Read the model definition and answer for the solid it produces. Units are mm, in the model's axes. Round coordinates to 2 decimals unless told otherwise and drop trailing zeros. Write each loop counter-clockwise with the first axis right and the second up, starting at its lowest first coordinate (ties: lowest second). Pieces come first, ordered by that corner, then holes. Notation, with made-up numbers: (73, -10.5) - (91, -10.5) arc R26 cw to (91, 12.5) - close; hole circle Ø4 at (61, -16.75). An arc over 180 degrees is marked (long way). Use one line per item in the form item = value. Start each with the question number.
1) The part is cut by section B-B, the plane x = -173.5. Give the vertices of the cut face in (y, z).
2) The part is cut by section A-A, the plane z = 3.2. Give the vertices of the cut face in (x, y), plus the area to 3 significant figures.
3) Consider line 1 along Y through (x, z) = (-39, 3.3); line 2 along X through (y, z) = (35.5, 2.45); line 3 along Y through (x, z) = (-174.5, 3.3). Determine where each line is inside the solid, lowest interval first. Write a range as from..to.
4) Each of these flat-tipped pins is pushed along its axis until it touches: pin 1 (0.6 mm diameter, centred on y = 54, z = 3.5, fed in from +X); pin 2 (0.6 mm diameter, centred on x = -68, z = 3.5, fed in from +Y). Where does it stop, or does it pass through?
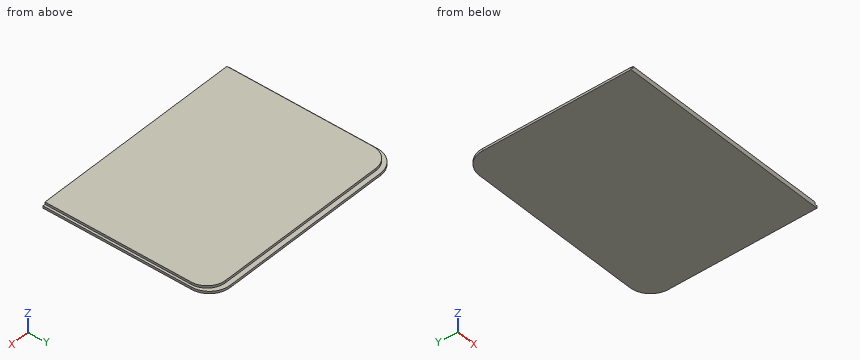
Autodesk Fusion 360 part; units mm, degrees
sketch "Sketch1" plane through (0, 0, 0) normal (0, 0, 1) x (1, 0, 0)
  line L0 (0, 0) -> (-187, 0)
  line L1 (-187, 0) -> (-187, 128)
  line L2 (-169, 146) -> (-18, 146)
  line L3 (0, 128) -> (0, 0)
  arc A0 (0, 128) -> (-18, 146) centre (-18, 128) ccw
  arc A1 (-169, 146) -> (-187, 128) centre (-169, 128) ccw
  line L4 (-185, 2) -> (-185, 126)
  line L5 (-2, 126) -> (-2, 2)
  line L6 (-185, 2) -> (-185, 0)
  line L7 (-2, 2) -> (-2, 0)
  line L8 (-169, 142) -> (-18, 142)
  arc A2 (-169, 142) -> (-185, 126) centre (-169, 126) ccw
  arc A3 (-2, 126) -> (-18, 142) centre (-18, 126) ccw
  point P0 (0, 146)
  dimension "d1" = 187
  dimension "d2" = 146
  dimension "d3" = 18
  dimension "d4" = 18
extrude "Extrude1" add sketch "Sketch1" along normal blind 4 contours L0 L4 L5 L6 L7 L8 A2 A3
extrude "Extrude2" add sketch "Sketch1" along normal blind 2 contours L0 L1 L2 L3 A0 A1 L4 L5 L6 L7 L8 A2 A3
Geometry results:
q1.outline = (0, 0) - (145.43, 0) - (145.43, 2) - (141.35, 2) - (141.35, 4) - (0, 4) - close
q2.outline = (-185, 0) - (-2, 0) - (-2, 126) arc R16 ccw to (-18, 142) - (-169, 142) arc R16 ccw to (-185, 126) - close
q2.area = 25,900 mm2
q3.line_1 = 0..142
q3.line_2 = -185..-2
q3.line_3 = 0..141.02
q4.pin_1 = -2
q4.pin_2 = 142
